Here's how the part is built. I have some questions about the finished solid (model axes, mm). A direction names the side the tool comes from. Round coordinates to 2 decimals unless told otherwise and drop trailing zeros. Order: outer loops, then holes, each group sorted by start corner. A loop starts at its lowest first (then second) coordinate and runs counter-clockwise, first axis right, second up. Notation, with made-up numbers: M 76,-31.75 L 134,-31.75 A11 cw 134,-16.75 Z; hole C 44,-6 d8. An arc over 180 degrees is marked long. Write item = value, one per line. Start each with the question number.
Item 1: I want a section at B-B, the plane y = 2.6. List the corners of the cut face in (x, z) for me, plus the area to 3 significant figures.
Item 2: For faces 1 (the face through (2, 3, 32)), 2 (the face through (3.05, 2.7, 33.5)), 3 (the face through (1.55, 2, 9)), which set-ups out of +Z, -Z, +X, -X, +Y, -Y let a thin tool reach every point of the face, with its end or its side?
Item 3: I want a section at A-A, the plane z = 11. List the corners of the cut face in (x, y) for me, plus the area to 3 significant figures.
Item 4: I want a section at C-C, the plane x = 15. List the corners of the cut face in (y, z) for me.
Item 5: We'd pull the mould along X, two halves only. Please class faces 4 (the face through (11, 1.5, 19)), 5 (the face through (28.4, 0.76, 37.93)), 6 (the face through (1.55, 2, 34)), 7 (the face through (14, 1, 0)): pulls with the +X half, pulls with the -X half, needs draft (parallel to the pull), parting line crosses it, or undercut.
Item 6: I'm going to push flat-ended pins straight in: P1, Ø3, axis at x = 26, z = 3.5, coming from the +Y side; P2, Ø2, axis at x = 20, y = 3, coming from the -Z side; P3, Ø1.5, axis at x = 16.5, y = 4, coming from the +Z side. Where does each tip first touch, or does it pass through?
Item 7: Please list where these lines run through material, in increasing order: L1, parallel to Z at x = 8.25, y = 2.5; L2, parallel to X at y = 1.85, z = 7; L3, parallel to Z at x = 3, y = 2.95.
Item 8: I want a section at D-D, the plane z = 28. List the corners of the cut face in (x, y) for me, plus the area to 4 significant figures.
```python
from build123d import *

# Parameters (mm, degrees)
SKETCH_1_W          = 29
SKETCH_1_H          = 38.5
EXTRUDE_2_DEPTH     = 4.5
SKETCH_3_W          = 29
SKETCH_3_H          = 38.5
SKETCH_3_W_2        = 25.9
SKETCH_3_H_2        = 35.3
CUT_EXTRUDE_1_DEPTH = 3
SKETCH_4_W          = 22.9
SKETCH_4_H          = 32.3
CUT_EXTRUDE_2_DEPTH = 3
SKETCH_5_W          = 17.9
SKETCH_5_H          = 1.5
CUT_EXTRUDE_3_DEPTH = 1
SKETCH_6_W          = 1.5
SKETCH_6_H          = 27.3
CUT_EXTRUDE_5_DEPTH = 1.5
FILLET_1_R          = 2
FILLET_5_R          = 0.5
SKETCH_8_W          = 17.9
SKETCH_8_H          = 1.5
EXTRUDE_7_DEPTH     = 0.2
FILLET_6_R          = 0.5
SKETCH_10_W         = 1.5
SKETCH_10_H         = 11
CUT_EXTRUDE_6_DEPTH = 1.5


with BuildPart() as part:
    # 草图1 → 凸台-拉伸2 (new body)
    with BuildSketch(Plane(origin=(0, 0, 0), x_dir=(1, 0, 0), z_dir=(0, 1, 0))):
        with Locations((14.5, -19.25)):
            Rectangle(SKETCH_1_W, SKETCH_1_H)
    extrude(amount=EXTRUDE_2_DEPTH)

    # 草图3 → 切除-拉伸1 (cut)
    with BuildSketch(Plane(origin=(0, 4.5, 0), x_dir=(1, 0, 0), z_dir=(0, 1, 0))):
        with Locations((14.5, -19.25)):
            Rectangle(SKETCH_3_W, SKETCH_3_H)
        with Locations((14.5, -19.25)):
            Rectangle(SKETCH_3_W_2, SKETCH_3_H_2, mode=Mode.SUBTRACT)
    extrude(amount=-CUT_EXTRUDE_1_DEPTH, mode=Mode.SUBTRACT)

    # 草图4 → 切除-拉伸2 (cut)
    with BuildSketch(Plane(origin=(0, 4.5, 0), x_dir=(1, 0, 0), z_dir=(0, 1, 0))):
        with Locations((14.5, -19.25)):
            Rectangle(SKETCH_4_W, SKETCH_4_H)
    extrude(amount=-CUT_EXTRUDE_2_DEPTH, mode=Mode.SUBTRACT)

    # 草图5 → 切除-拉伸3 (cut)
    with BuildSketch(Plane(origin=(0, 4.5, 0), x_dir=(1, 0, 0), z_dir=(0, 1, 0))):
        with Locations((14.5, -2.35)):
            Rectangle(SKETCH_5_W, SKETCH_5_H)
    extrude(amount=-CUT_EXTRUDE_3_DEPTH, mode=Mode.SUBTRACT)

    # 草图6 → 切除-拉伸5 (cut)
    with BuildSketch(Plane(origin=(0, 4.5, 0), x_dir=(1, 0, 0), z_dir=(0, 1, 0))):
        with Locations((2.3, -19.25)):
            Rectangle(SKETCH_6_W, SKETCH_6_H)
        with Locations((26.7, -19.25)):
            Rectangle(SKETCH_6_W, SKETCH_6_H)
    extrude(amount=-CUT_EXTRUDE_5_DEPTH, mode=Mode.SUBTRACT)

    # 圆角1
    fillet_1_edges = [part.edges().sort_by_distance(p)[0] for p in [
        (0, 0.75, 0),
        (29, 0.75, 0),
        (29, 0.75, 38.5),
        (0, 0.75, 38.5),
    ]]
    fillet(fillet_1_edges, radius=FILLET_1_R)

    # 圆角5
    fillet_5_edges = [part.edges().sort_by_distance(p)[0] for p in [
        (1.55, 3, 1.6),
        (27.45, 3, 1.6),
        (27.45, 3, 36.9),
        (1.55, 3, 36.9),
    ]]
    fillet(fillet_5_edges, radius=FILLET_5_R)

    # 草图8 → 凸台-拉伸7 (add)
    with BuildSketch(Plane(origin=(0, 4.5, 0), x_dir=(1, 0, 0), z_dir=(0, 1, 0))):
        with Locations((14.5, -36.15)):
            Rectangle(SKETCH_8_W, SKETCH_8_H)
    extrude(amount=EXTRUDE_7_DEPTH)

    # 圆角6
    fillet_6_edges = [part.edges().sort_by_distance(p)[0] for p in [
        (27.45, 4.5, 34.65),
        (25.2, 4.5, 1.6),
        (27.303553391, 4.5, 1.746446609),
        (1.55, 4.5, 3.85),
        (1.696446609, 4.5, 1.746446609),
        (3.8, 4.5, 36.9),
        (27.303553391, 4.5, 36.753553391),
        (1.696446609, 4.5, 36.753553391),
        (25.2, 4.5, 36.9),
        (3.8, 4.5, 1.6),
        (1.55, 4.5, 34.65),
        (27.45, 4.5, 3.85),
    ]]
    fillet(fillet_6_edges, radius=FILLET_6_R)

    # 草图10 → 切除-拉伸6 (cut)
    with BuildSketch(Plane(origin=(0, 3, 0), x_dir=(1, 0, 0), z_dir=(0, 1, 0))):
        with Locations((2.3, -24.9)):
            Rectangle(SKETCH_10_W, SKETCH_10_H)
    extrude(amount=-CUT_EXTRUDE_6_DEPTH, mode=Mode.SUBTRACT)


solid = part.part
```
Filled in:
q1.outline = M 1.55,2.1 A0.5 ccw 2.05,1.6 L 26.95,1.6 A0.5 ccw 27.45,2.1 L 27.45,36.4 A0.5 ccw 26.95,36.9 L 2.05,36.9 A0.5 ccw 1.55,36.4 L 1.55,30.4 L 3.05,30.4 L 3.05,35.4 L 25.95,35.4 L 25.95,3.1 L 3.05,3.1 L 3.05,19.4 L 1.55,19.4 Z
q1.area = 158 mm^2
q2.face_1 = +X, -X, +Y
q2.face_2 = +Y
q2.face_3 = +Z, -Z, -X, +Y
q3.outline = M 0,0 L 29,0 L 29,1.5 L 27.45,1.5 L 27.45,3 L 25.95,3 L 25.95,1.5 L 3.05,1.5 L 3.05,3 L 1.55,3 L 1.55,1.5 L 0,1.5 Z
q3.area = 48.0 mm^2
q4.outline = M 0,0 L 1.5,0 L 1.5,1.6 L 3.5,1.6 L 3.5,3.1 L 1.5,3.1 L 1.5,35.4 L 4.7,35.4 L 4.7,36.9 L 1.5,36.9 L 1.5,38.5 L 0,38.5 Z
q5.face_4 = undercut
q5.face_5 = pulls with the +X half
q5.face_6 = pulls with the -X half
q5.face_7 = needs draft
q6.P1 = 4.5
q6.P2 = 1.6
q6.P3 = 36.9
q7.L1 = 1.6 to 3.1, 35.4 to 36.9
q7.L2 = 1.55 to 3.05, 25.95 to 27.45
q7.L3 = 1.6 to 19.4, 30.4 to 36.9
q8.outline = M 0,0 L 29,0 L 29,1.5 L 27.45,1.5 L 27.45,3 L 25.95,3 L 25.95,1.5 L 0,1.5 Z
q8.area = 45.75 mm^2
